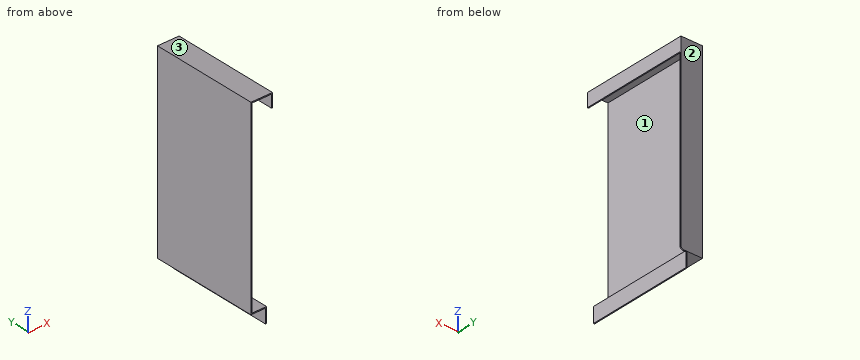
```python
from build123d import *

# Parameters (mm, degrees)
F4_DEPTH = 2


with BuildPart() as f2:
    # F2: sweep along a path in F1
    with BuildLine(Plane.XY) as f2_path:
        Line((0, 0), (0, 198))
    # F0 (on Front) → F2 (sweep)
    with BuildSketch(Plane.XZ):
        Polygon((40, 0), (0, 0), (0, -350), (27, -350), (27, -376), (29, -376), (29, -348), (2, -348), (2, -2), (38, -2), (38, -25), (40, -25), align=None)
    sweep(path=f2_path.line)

    # F3 (on face) → F4 (join)
    with BuildSketch(Plane(origin=(0, 198, 0), x_dir=(-1, 0, 0), z_dir=(0, 1, 0))):
        with BuildLine():
            Line((-27, -350), (0, -350))
            Line((0, -350), (0, 0))
            Line((0, 0), (-40, 0))
            Line((-40, 0), (-40, -25))
            Line((-40, -25), (-40, -345))
            ThreePointArc((-40, -345), (-38.5355339059, -348.5355339059), (-35, -350))
            Line((-35, -350), (-29, -350))
            Line((-29, -350), (-27, -350))
        make_face()
    extrude(amount=F4_DEPTH)


solid = f2.part
```
Check sheet for the modelled part. Datum: model origin and axes. Units: mm. Face numbers are marked on the shaded views. Coordinates: 2 decimals unless noted, no trailing zeros. Loops run counter-clockwise (first coordinate to the right, second up) from the corner with the lowest first, then second, coordinate; pieces in that order, holes last.
1) Release check for a two-part mould opening along Z. For the marked faces 1, 2 and 3 record: released by +Z, released by -Z, zero draft, split by the parting line, or undercut.
2) Material ranges on probe 1 along Z at (x, y) = (18.5, 170); probe 2 along X at (y, z) = (174, -24); probe 3 along Z at (x, y) = (28, 129.5), recorded low to high.
3) Sectioned sample at C-C (z = -269). Record the boundary of the cut face in (x, y), and give its area (3 significant figures).
4) Gauge pin test, flat ends, axial feed: pin 1 (10.5 mm diameter, centred on x = 14.5, y = 110, fed in from -Z); pin 2 (2 mm diameter, centred on x = 35.5, z = -41.5, fed in from -Y); pin 3 (3 mm diameter, centred on y = 138, z = -322, fed in from +X). Record the tip position at first contact, or that the pin passes through.
5) Sectioned sample at B-B (y = 139.5). Record the boundary of the cut face in (x, z), and give its area (3 significant figures).
6) Sectioned sample at A-A (x = 19.5). Record the boundary of the cut face in (y, z).
Check sheet entries:
1. face 1: undercut
1. face 2: zero draft
1. face 3: released by +Z
2. probe 1: z = -350 to -348, -2 to 0
2. probe 2: x = 0 to 2, 38 to 40
2. probe 3: z = -376 to -348, -2 to 0
3. outline: (0, 0) - (2, 0) - (2, 198) - (40, 198) - (40, 200) - (0, 200) - close
3. area: 476 mm2
4. pin 1: stops at z = -350
4. pin 2: stops at y = 198
4. pin 3: stops at x = 2
5. outline: (0, -350) - (27, -350) - (27, -376) - (29, -376) - (29, -348) - (2, -348) - (2, -2) - (38, -2) - (38, -25) - (40, -25) - (40, 0) - (0, 0) - close
5. area: 928 mm2
6. outline: (0, -350) - (200, -350) - (200, 0) - (0, 0) - (0, -2) - (198, -2) - (198, -348) - (0, -348) - close
